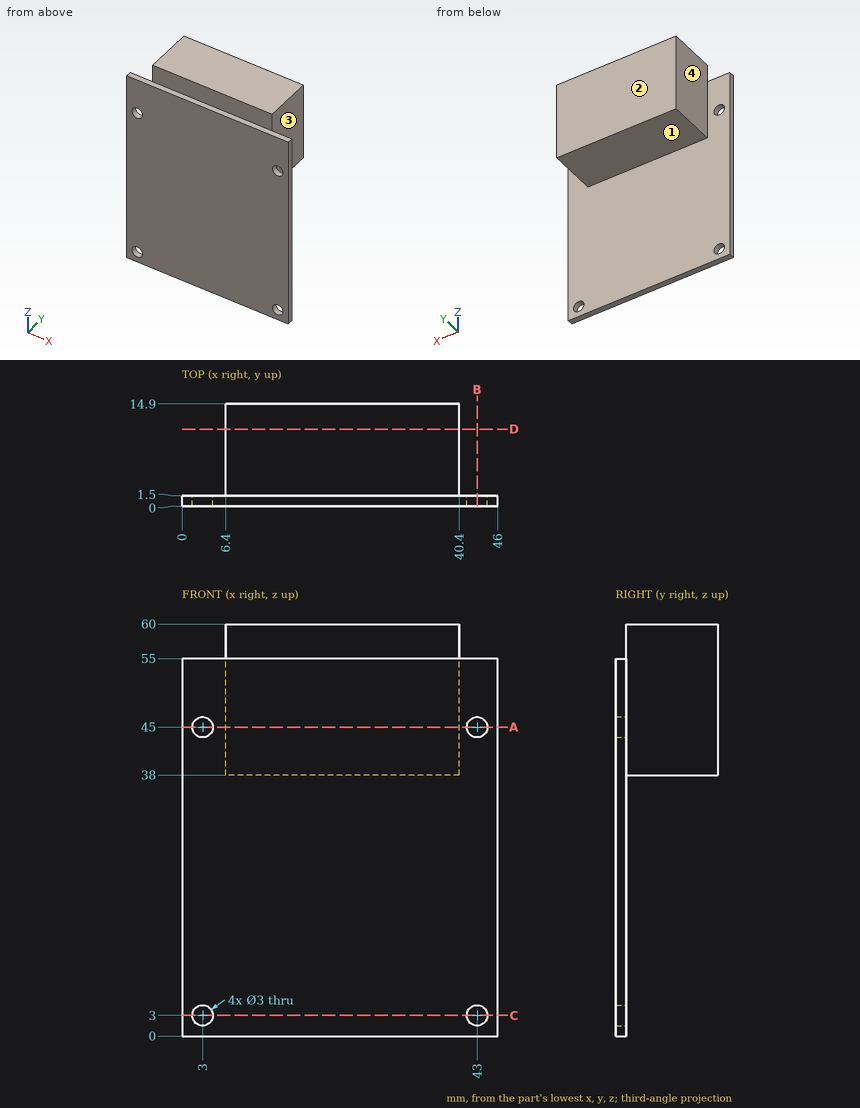
Verification items for this drawing (mm, ordinates from the low corner). A direction names the side the tool comes from. Round coordinates to 2 decimals unless told otherwise and drop trailing zeros. Write each loop counter-clockwise with the first axis right and the second up, starting at its lowest first coordinate (ties: lowest second). Pieces come first, ordered by that corner, then holes. Notation, with made-up numbers: (78.25, 41.5) - (136.25, 41.5) arc R30 cw to (136.25, 78.5) - close; hole circle Ø8 at (-35, 85). An arc over 180 degrees is marked (long way). Answer as a JSON object with one key per item and string values. Group by question number.
Q1. Thickness scan on line 1 (Z direction, x = 3, y = 0.6); line 2 (X direction, y = 0.6, z = 45); line 3 (Z direction, x = 34.5, y = 11.5). Record the ranges inside material, lowest first.
Q2. Section check C-C, the plane z = 3. Enter the section's corners in (x, y).
Q3. Section check B-B, the plane x = 43. Enter the section's corners in (y, z), plus the area to 3 significant figures.
Q4. Section check D-D, the plane y = 11.25. Enter the section's corners in (x, z).
Q5. Tool access check on the marked faces 1, 2, 3 and 4. Record the directions out of +Z, -Z, +X, -X, +Y, -Y that give a thin tool (end or side, any length) a straight path to the whole face; none if there is none.
Q6. Go/stop test with flat-tipped pins: pin 1 Ø3.5 at (x, z) = (3, 45) entering from +Y; pin 2 Ø5 at (y, z) = (4.5, 51) entering from +X; pin 3 Ø1.5 at (x, y) = (15.5, 5.5) entering from -Z; pin 4 Ø2.5 at (x, z) = (43, 3) entering from +Y. Record where each tip stops, or that it passes through.
Q7. Section check A-A, the plane z = 45. Enter the section's corners in (x, y), plus the area to 3 significant figures.
Found:
{
 "1": {"line 1": "z = 0 to 1.5, 4.5 to 43.5, 46.5 to 55", "line 2": "x = 0 to 1.5, 4.5 to 41.5, 44.5 to 46", "line 3": "z = 38 to 60"},
 "2": {"outline": "(0, 0) - (1.5, 0) - (1.5, 1.5) - (0, 1.5) - close; (4.5, 0) - (41.5, 0) - (41.5, 1.5) - (4.5, 1.5) - close; (44.5, 0) - (46, 0) - (46, 1.5) - (44.5, 1.5) - close"},
 "3": {"outline": "(0, 0) - (1.5, 0) - (1.5, 1.5) - (0, 1.5) - close; (0, 4.5) - (1.5, 4.5) - (1.5, 43.5) - (0, 43.5) - close; (0, 46.5) - (1.5, 46.5) - (1.5, 55) - (0, 55) - close", "area": "73.5 mm^2"},
 "4": {"outline": "(6.4, 38) - (40.4, 38) - (40.4, 60) - (6.4, 60) - close"},
 "5": {"face 1": "-Z, +X, -X, +Y", "face 2": "+Z, -Z, +X, -X, +Y", "face 3": "+Z, -Z, +X, +Y", "face 4": "+Z, -Z, -X, +Y"},
 "6": {"pin 1": "stops at y = 1.5", "pin 2": "stops at x = 40.4", "pin 3": "stops at z = 38", "pin 4": "passes through"},
 "7": {"outline": "(0, 0) - (1.5, 0) - (1.5, 1.5) - (0, 1.5) - close; (4.5, 0) - (41.5, 0) - (41.5, 1.5) - (40.4, 1.5) - (40.4, 14.9) - (6.4, 14.9) - (6.4, 1.5) - (4.5, 1.5) - close; (44.5, 0) - (46, 0) - (46, 1.5) - (44.5, 1.5) - close", "area": "516 mm^2"}
}
